from build123d import *

# Parameters (mm, degrees)
SKETCH1_W           = 34
SKETCH1_H           = 35.5
SKETCH1_R           = 2
BOSS_EXTRUDE1_DEPTH = 7.15


with BuildPart() as part:
    # Sketch1 → Boss-Extrude1 (new body)
    with BuildSketch(Plane.XY):
        with Locations((17, 17.75)):
            Rectangle(SKETCH1_W, SKETCH1_H)
        with Locations((4.431526268, 3.5)):
            Circle(SKETCH1_R, mode=Mode.SUBTRACT)
        with Locations((29.568473732, 3.5)):
            Circle(SKETCH1_R, mode=Mode.SUBTRACT)
        with Locations((29.568473732, 32)):
            Circle(SKETCH1_R, mode=Mode.SUBTRACT)
        with Locations((4.431526268, 32)):
            Circle(SKETCH1_R, mode=Mode.SUBTRACT)
    extrude(amount=BOSS_EXTRUDE1_DEPTH)

    # Sketch4 → Revolve2 (revolve)
    with BuildSketch(Plane(origin=(17, 0, 0), x_dir=(0, 0, -1), z_dir=(1, 0, 0))):
        Polygon((-7.15, 26.25), (-15.15, 26.25), (-17.829491924, 36.25), (-17.44582843, 36.75), (-14.766336506, 26.75), (-7.15, 26.75), align=None)
    revolve(axis=Axis((17, 17.75, 7.15), (0, 0, 1)))


solid = part.part
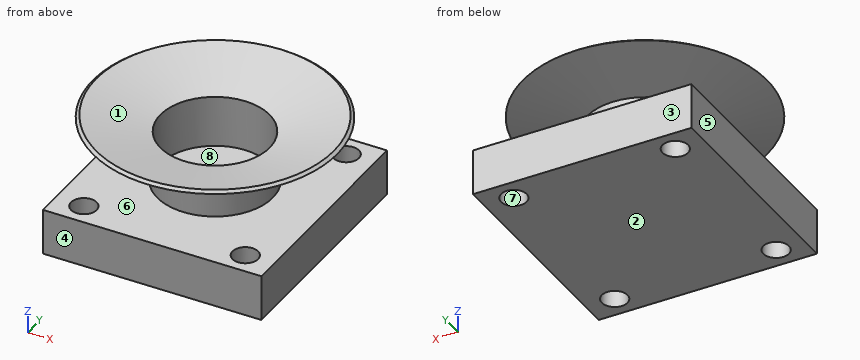
Input: part model. Units: mm. Frame: model coordinates. Face numbers are marked on the shaded views. A direction names the side the tool comes from. Coordinates: 2 decimals unless noted, no trailing zeros. Loops run counter-clockwise (first coordinate to the right, second up) from the corner with the lowest first, then second, coordinate; pieces in that order, holes last. Notation, with made-up numbers: (79.5, 54) -> (134.5, 54) arc R32 cw to (134.5, 89) -> close; hole circle Ø5 at (60.5, -39.75). An arc over 180 degrees is marked (long way). Write item = value, one per line. Start each with the question number.
Item 1: Cut plane A-A, the plane z = 4.25. Return loops of the section in (x, y).
Item 2: Material intervals for line 1 (Y direction, x = 29, z = 5.5); line 2 (Y direction, x = 17, z = 11.25); line 3 (X direction, y = 17.75, z = 10), sorted ascending.
Item 3: Mould query, pull axis Y, two halves, no side actions, for the marked faces 1, 2, 3 and 4. Classes: pulls with the +Y half, pulls with the -Y half, needs draft (parallel to the pull), parting line crosses it, or undercut.
Item 4: Cut plane B-B, the plane x = 17. Return loops of the section in (y, z).
Item 5: Cut plane D-D, the plane z = 12.5. Return loops of the section in (x, y), plus the area to 3 significant figures.
Item 6: First-contact query: P1, Ø3, axis at x = 4.43, y = 3.5, coming from the -Z side; P2, Ø18.5, axis at x = 21, y = 21, coming from the +Z side; P3, Ø5.5, axis at x = 10.5, z = 5, coming from the +Y side. Flat tips, straight axial feed; report the tip coordinate or a pass-through.
Item 7: Cut plane C-C, the plane y = 17.75. Return loops of the section in (x, z), plus the area to 3 significant figures.
Item 8: Reachability of the marked faces 5, 6, 7 and 8 from +Z, -Z, +X, -X, +Y, -Y: full face, straight path, thin tool, end or side. Return the list, or none.
Ans:
q1.outline = (0, 0) -> (34, 0) -> (34, 35.5) -> (0, 35.5) -> close; hole circle Ø4 at (4.43, 3.5); hole circle Ø4 at (4.43, 32); hole circle Ø4 at (29.57, 3.5); hole circle Ø4 at (29.57, 32)
q2.line_1 = 0 to 1.58, 5.42 to 30.08, 33.92 to 35.5
q2.line_2 = 8.75 to 9.25, 26.25 to 26.75
q2.line_3 = 8 to 8.5, 25.5 to 26
q3.face_1 = undercut
q3.face_2 = needs draft
q3.face_3 = pulls with the +Y half
q3.face_4 = pulls with the -Y half
q4.outline = (-1.25, 17.45) -> (8.75, 14.77) -> (8.75, 7.15) -> (0, 7.15) -> (0, 0) -> (35.5, 0) -> (35.5, 7.15) -> (26.75, 7.15) -> (26.75, 14.77) -> (36.75, 17.45) -> (36.25, 17.83) -> (26.25, 15.15) -> (26.25, 7.15) -> (9.25, 7.15) -> (9.25, 15.15) -> (-0.75, 17.83) -> close
q5.outline = circle Ø18 at (17, 17.75); hole circle Ø17 at (17, 17.75)
q5.area = 27.5 mm²
q6.P1 = 17.04
q6.P2 = 16.73
q6.P3 = 35.5
q7.outline = (-2, 17.45) -> (8, 14.77) -> (8, 7.15) -> (0, 7.15) -> (0, 0) -> (34, 0) -> (34, 7.15) -> (26, 7.15) -> (26, 14.77) -> (36, 17.45) -> (35.5, 17.83) -> (25.5, 15.15) -> (25.5, 7.15) -> (8.5, 7.15) -> (8.5, 15.15) -> (-1.5, 17.83) -> close
q7.area = 261 mm²
q8.face_5 = -Z, -X, +Y, -Y
q8.face_6 = none
q8.face_7 = -Z
q8.face_8 = +Z
